Autodesk Inventor part; units mm, degrees
ref_plane "YZ Plane" through (0, 0, 0) normal (1, 0, 0) x (0, 1, 0)
ref_plane "XZ Plane" through (0, 0, 0) normal (0, 1, 0) x (-1, 0, 0)
ref_plane "XY Plane" through (0, 0, 0) normal (0, 0, 1) x (1, 0, 0)
sketch "Sketch1" plane through (0, 0, 0) normal (0, 0, 1) x (1, 0, 0)
  circle A0 centre (0, 0) radius 1.5
  circle A1 centre (0, 0) radius 6
  line L0 (-19, 2.75) -> (-1.5, 2.75)
  line L1 (-1.5, 2.75) -> (-1.5, -2.75)
  line L2 (-1.5, -2.75) -> (-19, -2.75)
  line L3 (-19, -2.75) -> (-19, 2.75)
  line L4 (0, -8.4) -> (0, 8.4) construction
  line L5 (19, 2.75) -> (1.5, 2.75)
  line L6 (1.5, 2.75) -> (1.5, -2.75)
  line L7 (1.5, -2.75) -> (19, -2.75)
  line L8 (19, -2.75) -> (19, 2.75)
  point P0 (-1.5, 0)
  dimension "d0" = 3
  dimension "d1" = 12
  dimension "d2" = 17.5
  dimension "d3" = 5.5
extrude "Extrusion1" add sketch "Sketch1" along normal blind 2.5 contours L6 L7 A1 L2 L1 A0 | A0 L1 L0 A1 L5 L6 | L6 L5 A1 L7 | L1 L2 A1 L0 | L5 L8 L7 A1 | A1 L2 L3 L0
fillet "Fillet1" radius 2 4 edges at (-19, 2.75, 1.25) (-19, -2.75, 1.25) (19, 2.75, 1.25) (19, -2.75, 1.25)
chamfer "Chamfer6" distance 11.6666 distance2 1.5 1 edges at (-5.3327, 2.75, 1.25) measured on face at (-13.1109, 2.75, 0.8333)
chamfer "Chamfer7" distance 11.6666 distance2 1.5 1 edges at (5.3327, 2.75, 1.25) measured on face at (13.1109, 2.75, 0.8333)
chamfer "Chamfer8" distance 11.6666 distance2 1.5 1 edges at (-5.3327, -2.75, 1.25) measured on face at (-9.2218, -2.75, 1.6667)
chamfer "Chamfer9" distance 11.6666 distance2 1.5 1 edges at (5.3327, -2.75, 1.25) measured on face at (9.2218, -2.75, 0.8333)
sketch "Sketch3" plane through (0, 0, 2.5) normal (0, 0, 1) x (1, 0, 0)
  circle A0 centre (-7.5, 0) radius 1
  line L0 (-26.6, 0) -> (26.6, 0) construction
  circle A1 centre (-10.5, 0) radius 1
  circle A2 centre (-13.5, 0) radius 1
  circle A3 centre (-16.5, 0) radius 1
  line L1 (0, -8.4) -> (0, 8.4) construction
  circle A4 centre (7.5, 0) radius 1
  circle A5 centre (10.5, 0) radius 1
  circle A6 centre (13.5, 0) radius 1
  circle A7 centre (16.5, 0) radius 1
  point P0 (0, 0)
  dimension "d37" = 2
  dimension "d38" = 7.5
  dimension "d41" = 3
extrude "Extrusion3" cut sketch "Sketch3" against normal through all
sketch "Sketch4" plane through (0, 0, 0) normal (0, 0, -1) x (-1, 0, 0)
  circle A0 centre (0, 0) radius 1.5
  circle A1 centre (0, 0) radius 2.5
  circle A2 centre (0, 0) radius 4.25
  dimension "d48" = 5
  dimension "d49" = 8.5
extrude "Extrusion4" add sketch "Sketch4" along normal blind 3 contours A2
properties part number "ServoArm2"
Geometry check sheet. Reference: the model listing, model coordinates, mm. A direction names the side the tool comes from. Give positions to 0.01 mm unless a question says otherwise; leave off trailing zeros. Loops run counter-clockwise (first coordinate to the right, second up) from the corner with the lowest first, then second, coordinate; pieces in that order, holes last. Notation, with made-up numbers: M 36,-20 L 75,-20 A22 cw 75,-9 Z; hole C 72.5,16.5 d2. An arc over 180 degrees is marked long. Write item = value, one per line.
(1) Release check for a two-part mould opening along Y. For faces 3 (the face through (-10.654, 3.377, 1.233)), 4 (the face through (9.7, -0.6, 1.3)), 5 (the face through (10.654, -3.377, 1.233)) record: released by +Y, released by -Y, zero draft, split by the parting line, or undercut.
Answer below:
face_3 = released by +Y
face_4 = undercut
face_5 = released by -Y
(2) Sectioned sample at D-D, the plane x = -13.5. Record the cut outline in (y, z).
Answer below:
outline = M -3.1,0 L -1,0 L -1,2.5 L -3.1,2.5 Z; M 1,0 L 3.1,0 L 3.1,2.5 L 1,2.5 Z
(3) Sectioned sample at B-B, the plane z = 1.55. State how many separate pieces and enclosed holes the cut face has, plus the area to 3 significant figures.
Answer below:
separate_pieces = 1
enclosed_holes = 9
area = 252 mm2
(4) Material ranges on line 1 (Y direction, x = 0, z = -1); line 2 (Z direction, x = 5.5, y = -0.75); line 3 (Y direction, x = -0.5, z = -2), recorded low to high. Write a range as [from, to].
Answer below:
line_1 = [-4.25, -2.5], [2.5, 4.25]
line_2 = [0, 2.5]
line_3 = [-4.22, -2.45], [2.45, 4.22]
(5) Sectioned sample at A-A, the plane x = 0. Record the cut outline in (y, z), plus the area to 3 significant figures.
Answer below:
outline = M -6,0 L -4.25,0 L -4.25,-3 L -2.5,-3 L -2.5,0 L -1.5,0 L -1.5,2.5 L -6,2.5 Z; M 1.5,0 L 2.5,0 L 2.5,-3 L 4.25,-3 L 4.25,0 L 6,0 L 6,2.5 L 1.5,2.5 Z
area = 33.0 mm2
(6) Tool access check on faces 1 (the face through (2, 0, 0)), 2 (the face through (17.424, -0.383, 1.268)). Record the directions out of +Z, -Z, +X, -X, +Y, -Y that give a thin tool (end or side, any length) a straight path to the whole face; none if there is none.
Answer below:
face_1 = -Z
face_2 = +Z, -Z
(7) Gauge pin test, flat ends, axial feed: pin 1 Ø2.5 at (x, y) = (1, 0) entering from -Z; pin 2 Ø3 at (x, z) = (-5.5, 1) entering from -Y; pin 3 Ø3 at (x, z) = (13.5, 0) entering from +Y. Record the tip position at first contact, or that the pin passes through.
Answer below:
pin_1 = 0
pin_2 = -4.47
pin_3 = 3.24
